from build123d import *

# Parameters (mm, degrees)
FILLET3_SIZE       = 1
FILLET3_SIZE_2     = 3
CUT_EXTRUDE5_DEPTH = 0.5
CIRPATTERN3_COUNT  = 8


with BuildPart() as part:
    # Sketch2 → Revolve4 (revolve)
    with BuildSketch(Plane.XY, mode=Mode.PRIVATE) as revolve4_sk:
        with BuildLine():
            Line((-10.46, 0), (-10.46, -2))
            Line((-10.46, -2), (-7, -2))
            ThreePointArc((-7, -2), (-4.171572875, -3.171572875), (-3, -6))
            ThreePointArc((-3, -6), (-2.121320344, -8.121320344), (0, -9))
            Line((0, -9), (0, -6))
            ThreePointArc((0, -6), (-0.907428337, -2.553179648), (-3.394448725, 0))
            Line((-3.394448725, 0), (-10.46, 0))
        make_face()
    revolve(revolve4_sk.sketch.rotate(Axis((1, -9, 0), (0, 1, 0)), 270), axis=Axis((1, -9, 0), (0, 1, 0)))

    # Fillet3
    # an asymmetric fillet: 3, 1 mm, written as the material it takes off along each edge
    with BuildSketch(Plane(origin=(1, -2, 0), x_dir=(0, 0, -1), z_dir=(1, 0, 0))) as fillet3_piece_1:
        with BuildLine():
            Bezier((11.46, FILLET3_SIZE), (11.46, 0), (11.46 - FILLET3_SIZE_2, 0), weights=[1, 0.707106781, 1])
            Line((11.46 - FILLET3_SIZE_2, 0), (11.46, 0))
            Line((11.46, 0), (11.46, FILLET3_SIZE))
        make_face()
    revolve(axis=Axis((1, -2, 0), (0, 1, 0)), mode=Mode.SUBTRACT)

    # Sketch8 → Cut-Extrude5 (cut)
    with BuildSketch(Plane(origin=(0, 0, 0), x_dir=(1, 0, 0), z_dir=(0, 1, 0))):
        Polygon((0, 0), (18.255808177, 0), (16.586053461, 7.014284446), align=None)
    cut_extrude5 = extrude(amount=-CUT_EXTRUDE5_DEPTH, mode=Mode.SUBTRACT)

    # CirPattern3: Cut-Extrude5 ×8 about axis
    cirpattern3_axis = Axis((1, 0, 0), (0, 1, 0))
    for i in range(1, CIRPATTERN3_COUNT):
        add(cut_extrude5.rotate(cirpattern3_axis, i * 360 / CIRPATTERN3_COUNT), mode=Mode.SUBTRACT)


solid = part.part
Geometry check sheet. Reference: the model listing, model coordinates, mm. A direction names the side the tool comes from. Round coordinates to 2 decimals unless told otherwise and drop trailing zeros.
Item 1: Access from +Z, -Z, +X, -X, +Y, -Y to the whole of each face (thin tool, end or side, straight path). Record for faces 1 (the flat face through (-5.85, -0.25, 3.32)), 2 (the flat face through (-2.32, -0.25, -6.85)), 3 (the flat face through (8, -0.5, 4)), 4 (the flat face through (7.85, -0.25, -3.32)), 5 (the flat face through (-4, 0, -7)).
Item 2: Thickness scan on line 1 (X direction, y = -0.25, z = 4.75); line 2 (X direction, y = -8.25, z = 0.75); line 3 (X direction, y = -6.95, z = 0). Record the ranges inside material, lowest first.
Item 3: Gauge pin test, flat ends, axial feed: pin 1 (2 mm diameter, centred on x = -7.5, y = -1.5, fed in from -Z); pin 2 (2 mm diameter, centred on x = 8, z = 4.5, fed in from +Y); pin 3 (1 mm diameter, centred on y = -6.5, z = -3.5, fed in from -X); pin 4 (1.8 mm diameter, centred on x = 1, z = 0, fed in from -Y). Record the tip position at first contact, or that the pin passes through.
Item 4: Mould release check, pull along Z, two halves, no side actions. Record for faces 6 (the flat face through (6.3, -0.2, 5.3)), 7 (the flat face through (3, 0, -9)), 8 (the flat face through (4.32, -0.25, 6.85)): pulls with the +Z half, pulls with the -Z half, needs draft (parallel to the pull), parting line crosses it, or undercut.
Answer sheet:
1. face 1: -X, +Y
1. face 2: -Z, +Y
1. face 3: +Y
1. face 4: +X, +Y
1. face 5: +Z, -Z, +X, -X, +Y
2. line 1: x = -9.23 to -3.75, -0.51 to 1, 3.43 to 5.75
2. line 2: x = -1.89 to 0.34, 1.66 to 3.89
2. line 3: x = -2.85 to 0, 2 to 4.85
3. pin 1: stops at z = -8.57
3. pin 2: stops at y = -0.5
3. pin 3: stops at x = -1.59
3. pin 4: passes through
4. face 6: undercut
4. face 7: needs draft
4. face 8: pulls with the +Z half
